Geometry check sheet. Reference: drawing and pictorial views, mm from the part's lowest x, y, z. Give positions to 0.01 mm unless a question says otherwise; leave off trailing zeros. Write each loop counter-clockwise with the first axis right and the second up, starting at its lowest first coordinate (ties: lowest second). Pieces come first, ordered by that corner, then holes. Notation, with made-up numbers: M 51.5,43.5 L 73.5,43.5 A19 ccw 73.5,80.5 Z; hole C -0.5,16 d10. An arc over 180 degrees is marked long. Write item = value, one per line. Start each with the question number.
1) Mould release check, pull along Y, two halves, no side actions. Record for the marked faces 1, 2, 3 and 4: released by +Y, released by -Y, zero draft, split by the parting line, or undercut.
2) Cross-section at A-A, the plane y = 16. Record the cut outline in (x, z).
3) Go/stop test with flat-tipped pins: pin 1 (0.7 mm diameter, centred on x = 3, y = 22, fed in from -Z); pin 2 (0.7 mm diameter, centred on x = 3.5, y = 16, fed in from +Z). Record where each tip stops, or that it passes through.
4) Scan lines: line 1 along Y through (x, z) = (5.5, 56); line 2 along Y through (x, z) = (5.25, 47.5) (1 decimal); line 3 along Z through (x, y) = (0.75, 18). Record each from-to range of solid material in increasing order. Write a range as [from, to].
5) Cross-section at B-B, the plane z = 56. Record the cut outline in (x, y).
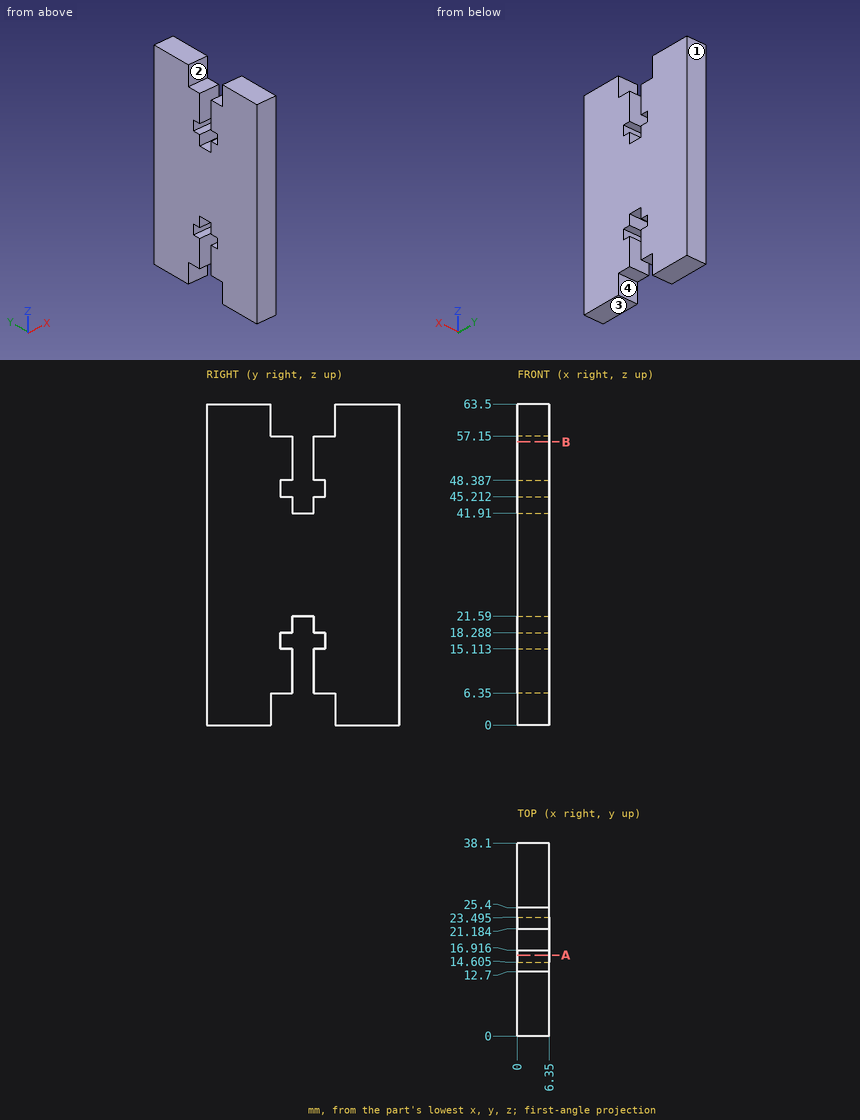
Reply:
q1.face_1 = released by +Y
q1.face_2 = undercut
q1.face_3 = zero draft
q1.face_4 = undercut
q2.outline = M 0,6.35 L 6.35,6.35 L 6.35,15.11 L 0,15.11 Z; M 0,18.29 L 6.35,18.29 L 6.35,45.21 L 0,45.21 Z; M 0,48.39 L 6.35,48.39 L 6.35,57.15 L 0,57.15 Z
q3.pin_1 = 6.35
q3.pin_2 = 57.15
q4.line_1 = [0, 16.92], [21.18, 38.1]
q4.line_2 = [0, 14.6], [23.5, 38.1]
q4.line_3 = [21.59, 41.91]
q5.outline = M 0,0 L 6.35,0 L 6.35,16.92 L 0,16.92 Z; M 0,21.18 L 6.35,21.18 L 6.35,38.1 L 0,38.1 Z
